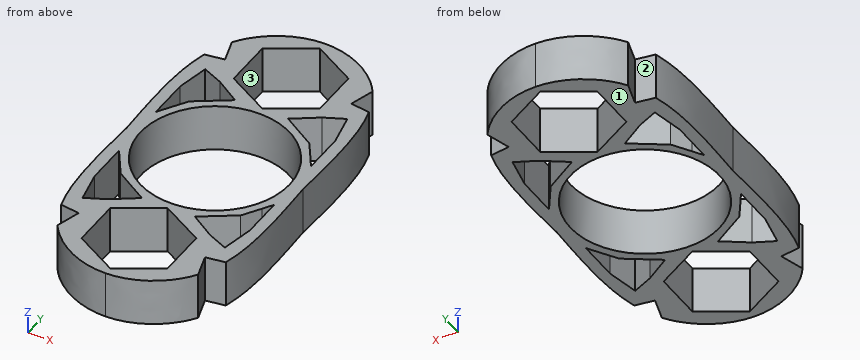
```python
from build123d import *

# Parameters (mm, degrees)
F0_R     = 11.1
F1_DEPTH = 7


with BuildPart() as f1:
    # F0 (on Top) → F1 (new body)
    with BuildSketch(Plane.XY):
        with BuildLine():
            add(Edge.make_bspline(
                [(0, 28.1878467649), (3.8763035152, 28.2040634856), (8.0688480164, 26.1116467562), (10.4658603604, 22.4543227052)],
                knots=[0, 0, 0, 0, 0.4129058091, 0.4129058091, 0.4129058091, 0.4129058091], degree=3))
            add(Edge.make_bspline(
                [(0, 28.1878467649), (-3.8763035152, 28.2040634856), (-8.0688480164, 26.1116467562), (-10.4658603604, 22.4543227052)],
                knots=[0, 0, 0, 0, 0.4129058091, 0.4129058091, 0.4129058091, 0.4129058091], degree=3))
            Line((-10.4658603604, 22.4543227052), (-9.3901595101, 18.8373755664))
            Line((-9.3901595101, 18.8373755664), (-12.2452968513, 18.429759182))
            add(Edge.make_bspline(
                [(-12.2452968513, 18.429759182), (-13.6777081897, 13.4016693255), (-13.3470218498, 6.8416931392), (-13.0910407752, 0)],
                knots=[0.5468406746, 0.5468406746, 0.5468406746, 0.5468406746, 1, 1, 1, 1], degree=3))
            add(Edge.make_bspline(
                [(-12.2452968513, -18.429759182), (-13.6777081897, -13.4016693255), (-13.3470218498, -6.8416931392), (-13.0910407752, 0)],
                knots=[0.5468406746, 0.5468406746, 0.5468406746, 0.5468406746, 1, 1, 1, 1], degree=3))
            Line((-12.2452968513, -18.429759182), (-9.3901595101, -18.8373755664))
            Line((-9.3901595101, -18.8373755664), (-10.4658603604, -22.4543227052))
            add(Edge.make_bspline(
                [(0, -28.1878467649), (-3.8763035152, -28.2040634856), (-8.0688480164, -26.1116467562), (-10.4658603604, -22.4543227052)],
                knots=[0, 0, 0, 0, 0.4129058091, 0.4129058091, 0.4129058091, 0.4129058091], degree=3))
            add(Edge.make_bspline(
                [(0, -28.1878467649), (3.8763035152, -28.2040634856), (8.0688480164, -26.1116467562), (10.4658603604, -22.4543227052)],
                knots=[0, 0, 0, 0, 0.4129058091, 0.4129058091, 0.4129058091, 0.4129058091], degree=3))
            Line((10.4658603604, -22.4543227052), (9.3901595101, -18.8373755664))
            Line((9.3901595101, -18.8373755664), (12.2452968513, -18.429759182))
            add(Edge.make_bspline(
                [(12.2452968513, -18.429759182), (13.6777081897, -13.4016693255), (13.3470218498, -6.8416931392), (13.0910407752, 0)],
                knots=[0.5468406746, 0.5468406746, 0.5468406746, 0.5468406746, 1, 1, 1, 1], degree=3))
            add(Edge.make_bspline(
                [(12.2452968513, 18.429759182), (13.6777081897, 13.4016693255), (13.3470218498, 6.8416931392), (13.0910407752, 0)],
                knots=[0.5468406746, 0.5468406746, 0.5468406746, 0.5468406746, 1, 1, 1, 1], degree=3))
            Line((12.2452968513, 18.429759182), (9.3901595101, 18.8373755664))
            Line((9.3901595101, 18.8373755664), (10.4658603604, 22.4543227052))
        make_face()
        Polygon((-11.5394731984, -4.7315182164), (-10.5750951916, -6.2584495172), (-8.9276162907, -8.8301226497), (-3.9449990727, -12.0045328513), (-7.601597812, -14.4154764712), (-10.5750951916, -15.7816782594), (-11.5394731984, -10.9999720007), align=None, mode=Mode.SUBTRACT)
        Polygon((-6.4, -23.2869711138), (-6.4, -15.8968876682), (0, -12.2018459454), (6.4, -15.8968876682), (6.4, -23.2869711138), (0, -26.9820128367), align=None, mode=Mode.SUBTRACT)
        Polygon((8.9276162907, -8.8301226497), (10.5750951916, -6.2584495172), (11.5394731984, -4.7315182164), (11.5394731984, -10.9999720007), (10.5750951916, -15.7816782594), (7.601597812, -14.4154764712), (3.9449990727, -12.0045328513), align=None, mode=Mode.SUBTRACT)
        Polygon((-8.9276162907, 8.8301226497), (-10.5750951916, 6.2584495172), (-11.5394731984, 4.7315182164), (-11.5394731984, 10.9999720007), (-10.5750951916, 15.7816782594), (-7.601597812, 14.4154764712), (-3.9449990727, 12.0045328513), align=None, mode=Mode.SUBTRACT)
        Circle(F0_R, mode=Mode.SUBTRACT)
        Polygon((3.9449990727, 12.0045328513), (7.601597812, 14.4154764712), (10.5750951916, 15.7816782594), (11.5394731984, 10.9999720007), (11.5394731984, 4.7315182164), (10.5750951916, 6.2584495172), (8.9276162907, 8.8301226497), align=None, mode=Mode.SUBTRACT)
        Polygon((0, 26.9820128367), (6.4, 23.2869711138), (6.4, 15.8968876682), (0, 12.2018459454), (-6.4, 15.8968876682), (-6.4, 23.2869711138), align=None, mode=Mode.SUBTRACT)
    extrude(amount=F1_DEPTH)


solid = f1.part
```
Verification items for the finished model (mm, model axes). Face numbers are marked on the shaded views. Round coordinates to 2 decimals unless told otherwise and drop trailing zeros. Put each result on its own line as item: value. Start each with the question number.
(1) Depth check by flat-ended pin: pin 1 Ø1 at (y, z) = (-5, 5.5) entering from -X; pin 2 Ø3 at (y, z) = (-16.5, 4) entering from -X; pin 3 Ø1.5 at (x, z) = (-1.5, 4.5) entering from +Y. Enter the tip coordinate at first touch or a pass-through.
(2) Section check A-A (z = 5.25). State how many separate pieces and enclosed holes the cut face has, then the cut area to 3 significant figures.
(3) Material ranges on line 1 along Y through (x, z) = (0, 4); line 2 along Y through (x, z) = (-7.5, 6.75); line 3 along Y through (x, z) = (4.25, 5.5), recorded low to high.
(4) Draft check along Y on the marked faces 1, 2 and 3. Enter one of: +Y half, -Y half, draft (parallel to the pull), parting line (faces both ways), or undercut.
Completed:
1. pin 1: stops at x = -13.28
1. pin 2: stops at x = -12.94
1. pin 3: stops at y = 28.17
2. separate pieces: 1
2. enclosed holes: 7
2. area: 479 mm2
3. line 1: y = -28.19 to -26.98, -12.2 to -11.1, 11.1 to 12.2, 26.98 to 28.19
3. line 2: y = -25.61 to -14.35, -9.74 to -8.18, 8.18 to 9.74, 14.35 to 25.61
3. line 3: y = -27.4 to -24.53, -14.66 to -12.21, -11.81 to -10.25, 10.25 to 11.81, 12.21 to 14.66, 24.53 to 27.4
4. face 1: draft
4. face 2: undercut
4. face 3: undercut
